Autodesk Inventor part; units mm, degrees
ref_plane "YZ Plane" through (0, 0, 0) normal (1, 0, 0) x (0, 1, 0)
ref_plane "XZ Plane" through (0, 0, 0) normal (0, 1, 0) x (-1, 0, 0)
ref_plane "XY Plane" through (0, 0, 0) normal (0, 0, 1) x (1, 0, 0)
sketch "Sketch_1" plane through (0, 0, 0) normal (0, 0, 1) x (1, 0, 0)
  line L0 (5, 0) -> (-10.8, 0)
  line L1 (-10.8, 0) -> (-10.8, 5)
  line L2 (-10.8, 5) -> (-8, 5)
  line L3 (-8, 5) -> (-8, 3)
  line L4 (-8, 3) -> (0, 3)
  line L5 (0, 3) -> (0, 2)
  line L6 (0, 2) -> (4.5705, 2)
  line L7 (4.5705, 2) -> (5, 1.5705)
  line L8 (5, 1.5705) -> (5, 0)
  line L9 (5, 0) -> (-10.8, 0)
revolve "Revolution1" add sketch "Sketch_1" angle 360 about axis through (5, 0, 0) along (1, 0, 0)
thread "Thread1"
sketch "Sketch_2" plane through (-10.8, 0, 0) normal (-1, 0, 0) x (0, 1, 0)
  line L0 (-1.4434, 0) -> (-0.7217, -1.25)
  line L1 (-0.7217, -1.25) -> (0.7217, -1.25)
  line L2 (0.7217, -1.25) -> (1.4434, 0)
  line L3 (1.4434, 0) -> (0.7217, 1.25)
  line L4 (0.7217, 1.25) -> (-0.7217, 1.25)
  line L5 (-0.7217, 1.25) -> (-1.4434, 0)
extrude "Extrusion1" cut sketch "Sketch_2" against normal blind 2.5
sketch "Sketch_3" plane through (0, 0, 0) normal (0, 0, 1) x (1, 0, 0)
  line L0 (-7.5783, 0) -> (-8.3, 0)
  line L1 (-8.3, 0) -> (-8.3, 1.25)
  line L2 (-8.3, 1.25) -> (-7.5783, 0)
  line L3 (-7.5783, 0) -> (-8.3, 0)
revolve "Revolution2" cut sketch "Sketch_3" angle 360 about axis through (-7.5783, 0, 0) along (1, 0, 0)
properties part number "DBB4-8-5" material "스테인리스스틸"
The listing builds one solid part. Answer for the finished solid, in the listing's coordinates (mm). A direction names the side the tool comes from. Round coordinates to 2 decimals unless told otherwise and drop trailing zeros. Loops run counter-clockwise (first coordinate to the right, second up) from the corner with the lowest first, then second, coordinate; pieces in that order, holes last. Notation, with made-up numbers: M -28.5,-24 L 30.5,-24 A32 cw 30.5,7 Z; hole C 81.25,61.5 d2. An arc over 180 degrees is marked long. Write each question's results on one line, items separated by ' | '. Start each with the question number.
1) Determine the mould class of faces 1 (the cylindrical face through (-9.38, -1.08, -4.88)), 2 (the flat face through (-10, 0, -1.25)), 3 (the flat face through (-10.8, 1.04, -1.04)) for opening direction Z: pulls with the +Z half, pulls with the -Z half, needs draft (parallel to the pull), parting line crosses it, or undercut.
2) Straight lines are drawn through the part: probe 1 along X at (y, z) = (1, 4.25); probe 2 along X at (y, z) = (-2.25, 1.25); probe 3 along Z at (x, y) = (-6.5, 0). For each, find the intervals that lie inside material, in ascending order.
3) Each of these flat-tipped pins is pushed along its axis until it touches: pin 1 (4 mm diameter, centred on x = 3, z = -2.5, fed in from -Y); pin 2 (3 mm diameter, centred on x = -9, z = -3, fed in from +Y); pin 3 (3 mm diameter, centred on x = -1.5, y = -3.5, fed in from -Z). Where does it stop, or does it pass through?
4) Which of the six approach directions +Z, -Z, +X, -X, +Y, -Y give full straight-line access (tool end or side, diameter ignored) to faces 4 (the flat face through (5, 0, 0)), 5 (the flat face through (-9.57, -1.08, -0.63)), 6 (the flat face through (-8, 3.3, 0.1))?
5) Find section B-B on y = 2.25. Write down the section's boundary in (x, z).
6) Find section C-C on x = 3.5. Write down the section's boundary in (y, z), plus the area to 3 significant figures.
7) Find section A-A on x = -4.5. Write down the section's boundary in (y, z).
Final values:
1) face 1: parting line crosses it | face 2: undercut | face 3: needs draft
2) probe 1: -10.8 to -8 | probe 2: -10.8 to 0 | probe 3: -3 to 3
3) pin 1: y = -1.94 | pin 2: y = 4.77 | pin 3: z = -2.24
4) face 4: +Z, -Z, +X, +Y, -Y | face 5: -X | face 6: +X
5) outline: M -10.8,-4.47 L -8,-4.47 L -8,-1.98 L 0,-1.98 L 0,1.98 L -8,1.98 L -8,4.47 L -10.8,4.47 Z
6) outline: C 0,0 d4 | area: 12.6 mm²
7) outline: C 0,0 d6
